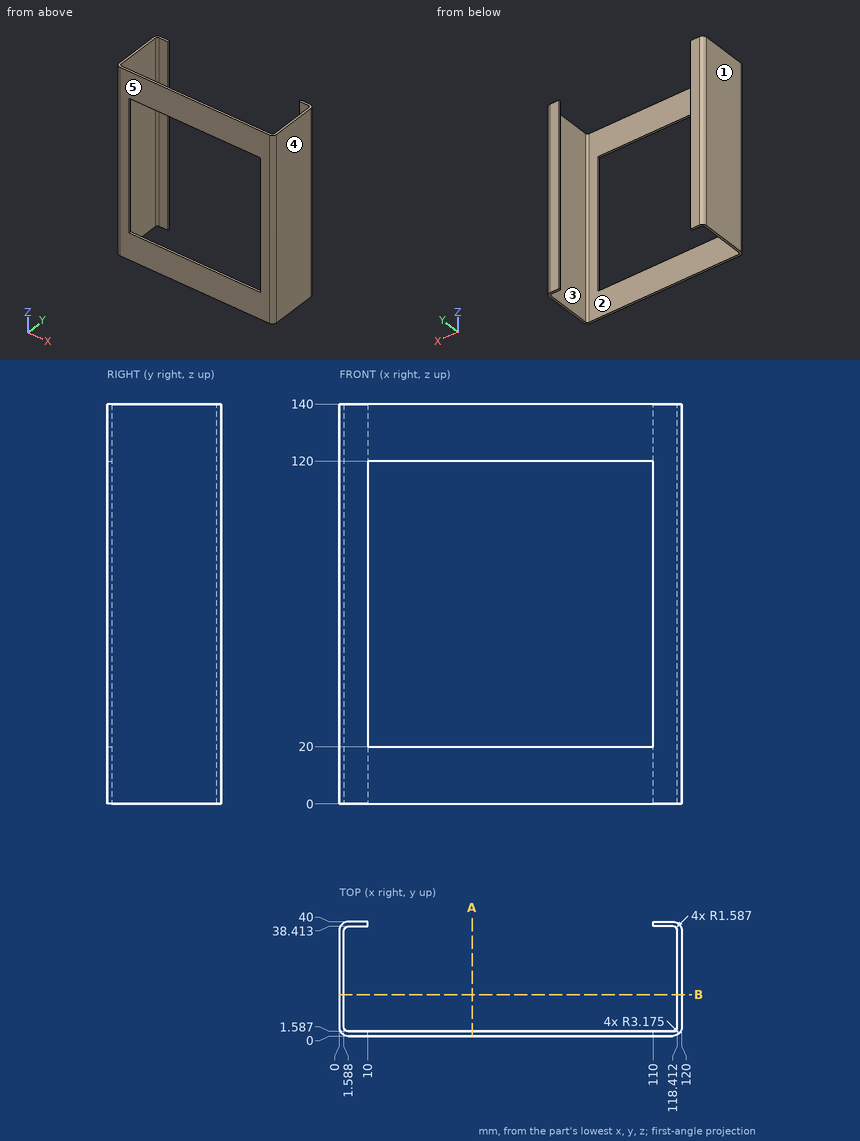
The drawing under review shows one solid part. Ordinate dimensions are in mm from its lowest x, y, z. A direction names the side the tool comes from. Give positions to 0.01 mm unless a question says otherwise; leave off trailing zeros. Write each loop counter-clockwise with the first axis right and the second up, starting at its lowest first coordinate (ties: lowest second). Pieces come first, ordered by that corner, then holes.
1. Tool access review of the marked faces 1 and 2: name each direction out of +Z, -Z, +X, -X, +Y, -Y from which nothing blocks a thin tool from reaching the whole face with its end or side.
2. Add section A-A, the plane x = 46.5. Write out the cut boundary in (y, z).
3. Wall thickness on L1, parallel to X at y = 16, z = 23; L2, parallel to Y at x = 8.5, z = 113; L3, parallel to Y at x = 38.5, z = 16: over which ranges is each line inside the solid? List them lowest first.
4. For P1, Ø0.5, axis at y = 39, z = 42.5, coming from the +X side; P2, Ø0.8, axis at y = 1, z = 53.5, coming from the -X side; P3, Ø1.7, axis at y = 0.5, z = 62, coming from the +X side, all flat-tipped, find the tip position at first contact; note any pin that passes through.
5. Add section B-B, the plane y = 14.5. Write out the cut boundary in (x, z).
6. Draft analysis for pull direction Y (two halves, no side actions). For the marked faces 3, 4 and 5, state which applies: +Y half, -Y half, draft (parallel to the pull), parting line (faces both ways), or undercut.
Worked answers:
1. face 1: +Z, -Z, -X, +Y, -Y
1. face 2: +Z, -Z
2. outline: (0, 0) - (1.59, 0) - (1.59, 20) - (0, 20) - close; (0, 120) - (1.59, 120) - (1.59, 140) - (0, 140) - close
3. L1: x = 0 to 1.59, 118.41 to 120
3. L2: y = 0 to 1.59, 38.41 to 40
3. L3: y = 0 to 1.59
4. P1: stops at x = 119.35
4. P2: stops at x = 0.54
4. P3: stops at x = 119.42
5. outline: (0, 0) - (1.59, 0) - (1.59, 140) - (0, 140) - close; (118.41, 0) - (120, 0) - (120, 140) - (118.41, 140) - close
6. face 3: undercut
6. face 4: draft
6. face 5: -Y half
